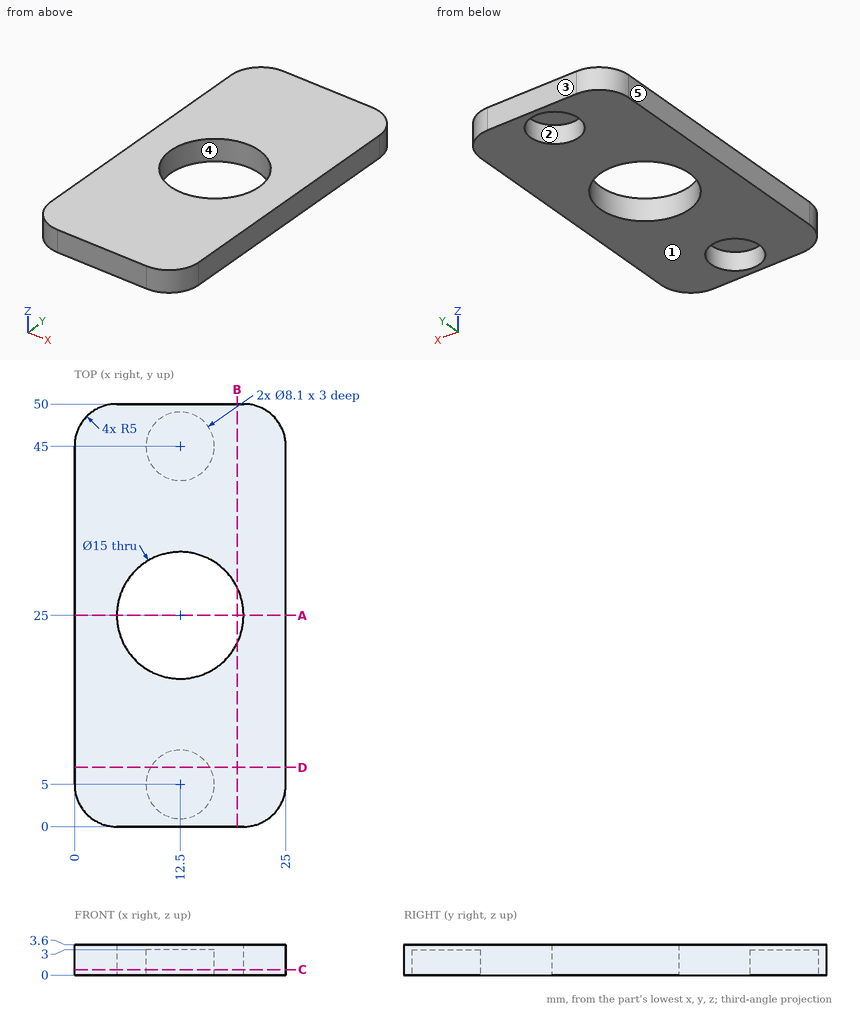
The figure shows three views and two pictorial views of one solid part (mm, origin at its lowest corner). Answer the questions. A direction names the side the tool comes from. Round coordinates to 2 decimals unless told otherwise and drop trailing zeros. Loops run counter-clockwise (first coordinate to the right, second up) from the corner with the lowest first, then second, coordinate; pieces in that order, holes last. Notation, with made-up numbers: M -6.5,9 L 31.5,9 A11 cw 31.5,27 Z; hole C 1,-20 d10. An arc over 180 degrees is marked long. Return JSON: item names as keys, results as strings.
Q1. Which of the six approach directions +Z, -Z, +X, -X, +Y, -Y give full straight-line access (tool end or side, diameter ignored) to the marked faces 1 and 2?
Results list:
{"face 1": "-Z, +X, -X, +Y, -Y", "face 2": "-Z"}
Q2. Find section C-C, the plane z = 0.65. Determine the outline of the cut face in (x, y), plus the area to 3 significant figures.
Results list:
{"outline": "M 0,5 A5 ccw 5,0 L 20,0 A5 ccw 25,5 L 25,45 A5 ccw 20,50 L 5,50 A5 ccw 0,45 Z; hole C 12.5,25 d15; hole C 12.5,5 d8.1; hole C 12.5,45 d8.1", "area": "949 mm2"}
Q3. Find section B-B, the plane x = 19.25. Determine the outline of the cut face in (y, z).
Results list:
{"outline": "M 0,0 L 21.73,0 L 21.73,3.6 L 0,3.6 Z; M 28.27,0 L 50,0 L 50,3.6 L 28.27,3.6 Z"}
Q4. This flat-tipped pin is pushed along its axis until it touches: pin 1 Ø4 at (x, y) = (12, 4) entering from -Z. Where does it stop, or does it pass through?
Results list:
{"pin 1": "stops at z = 3"}
Q5. Find the intervals of material crossed by line 1 along Y through (x, z) = (12.5, 0.85); line 2 along X through (y, z) = (5, 2.45); line 3 along Y through (x, z) = (16, 1.8), in increasing order. Write a range as from..to.
Results list:
{"line 1": "y = 0..0.95, 9.05..17.5, 32.5..40.95, 49.05..50", "line 2": "x = 0..8.45, 16.55..25", "line 3": "y = 0..2.96, 7.04..18.37, 31.63..42.96, 47.04..50"}
Q6. Find section D-D, the plane y = 7. Determine the outline of the cut face in (x, z), plus the area to 3 significant figures.
Results list:
{"outline": "M 0,0 L 8.98,0 L 8.98,3 L 16.02,3 L 16.02,0 L 25,0 L 25,3.6 L 0,3.6 Z", "area": "68.9 mm2"}
Q7. The mould has two halves that part along Y. Classify the marked faces 3, 4 and 5: released by +Y, released by -Y, zero draft, split by the parting line, or undercut.
Results list:
{"face 3": "released by +Y", "face 4": "undercut", "face 5": "zero draft"}
Q8. Find section A-A, the plane y = 25. Determine the outline of the cut face in (x, z), plus the area to 3 significant figures.
Results list:
{"outline": "M 0,0 L 5,0 L 5,3.6 L 0,3.6 Z; M 20,0 L 25,0 L 25,3.6 L 20,3.6 Z", "area": "36.0 mm2"}
